Here's the drawing with two shaded views (mm, measured from the low corner). I have some questions. Coordinates: 2 decimals unless noted, no trailing zeros. Loops run counter-clockwise (first coordinate to the right, second up) from the corner with the lowest first, then second, coordinate; pieces in that order, holes last. Notation, with made-up numbers: (28.25, 37) - (58.25, 37) arc R20 ccw to (58.25, 53) - close; hole circle Ø9 at (-19.75, -37.75). An arc over 180 degrees is marked (long way). One line per item, written item: value. Start each with the question number.
(1) If I drill on line 1 along Y through (x, z) = (19.5, 70.5); line 2 along X through (y, z) = (26, 29); line 3 along Y through (x, z) = (17, 34.5), over which ranges is the centre line in solid material (lowest first)? Write a range as from..to.
(2) If we mould it in two halves opening along X, with no side actions, what happens to the marked faces 1 and 2? For each: pulls with the +X half, pulls with the -X half, needs draft (parallel to the pull), parting line crosses it, or undercut.
(3) If we section it at B-B on z = 26: Write out the boundary of the cut face in (x, y).
(4) I'm going to push flat-ended pins straight in: P1, Ø6.5, axis at y = 19.61, z = 65.14, coming from the +X side; P2, Ø4, axis at x = 20.5, z = 89.5, coming from the +Y side; P3, Ø12, axis at x = 33.5, z = 64.5, coming from the -Y side; P4, Ø1.5, axis at y = 5.5, z = 67, coming from the +X side. Where does each tip first touch, or does it pass through?
(5) If we section it at C-C on y = 26: Write out the boundary of the cut face in (x, z), then the cut area to 3 significant figures.
(6) If we section it at A-A on x = 20: Write out the boundary of the cut face in (y, z), then the cut area to 4 significant figures.
(7) If we section it at D-D on y = 4: Write out the boundary of the cut face in (x, z), then the cut area to 3 significant figures.
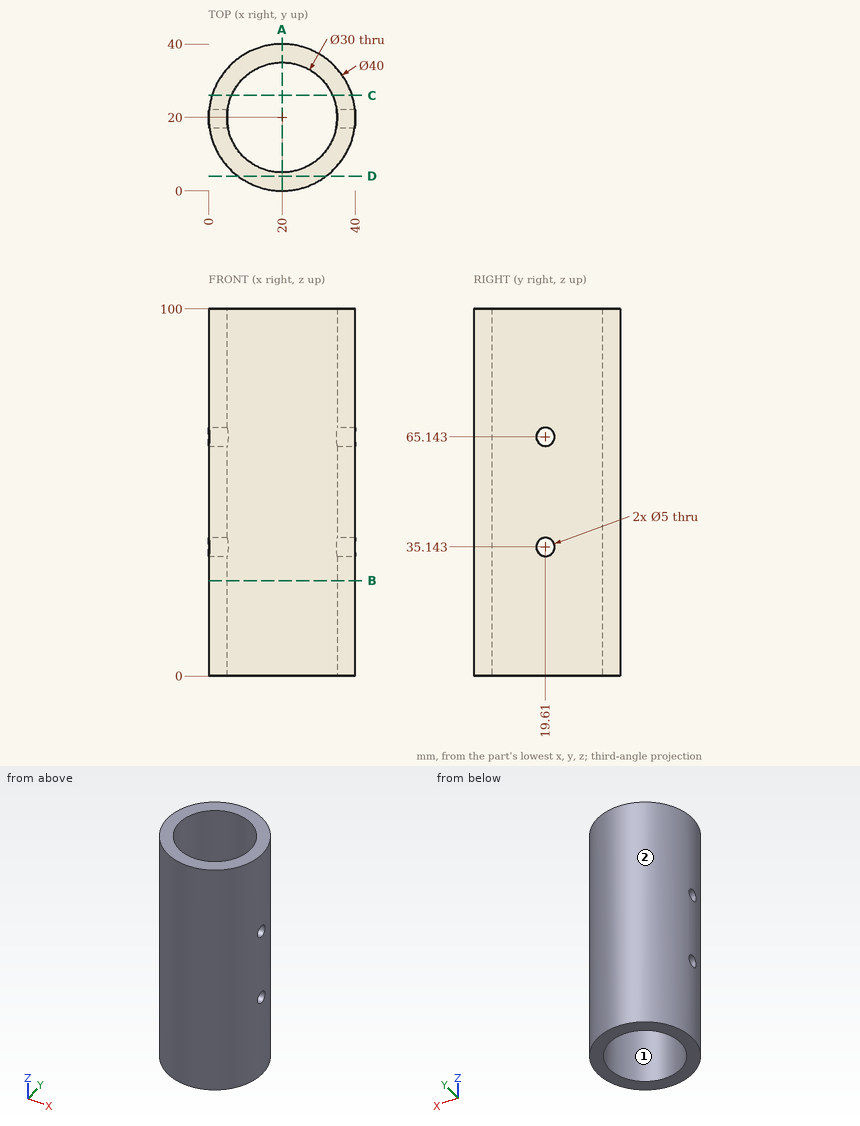
Values:
1. line 1: y = 0.01..5.01, 34.99..39.99
1. line 2: x = 0.92..6.25, 33.75..39.08
1. line 3: y = 0.23..5.3, 34.7..39.77
2. face 1: undercut
2. face 2: parting line crosses it
3. outline: circle Ø40 at (20, 20); hole circle Ø30 at (20, 20)
4. P1: stops at x = 40
4. P2: stops at y = 40
4. P3: stops at y = 1.46
4. P4: stops at x = 34.52
5. outline: (0.92, 0) - (6.25, 0) - (6.25, 100) - (0.92, 100) - close; (33.75, 0) - (39.08, 0) - (39.08, 100) - (33.75, 100) - close
5. area: 1,070 mm2
6. outline: (0, 0) - (5, 0) - (5, 100) - (0, 100) - close; (35, 0) - (40, 0) - (40, 100) - (35, 100) - close
6. area: 1,000 mm2
7. outline: (8, 0) - (32, 0) - (32, 100) - (8, 100) - close
7. area: 2,400 mm2
